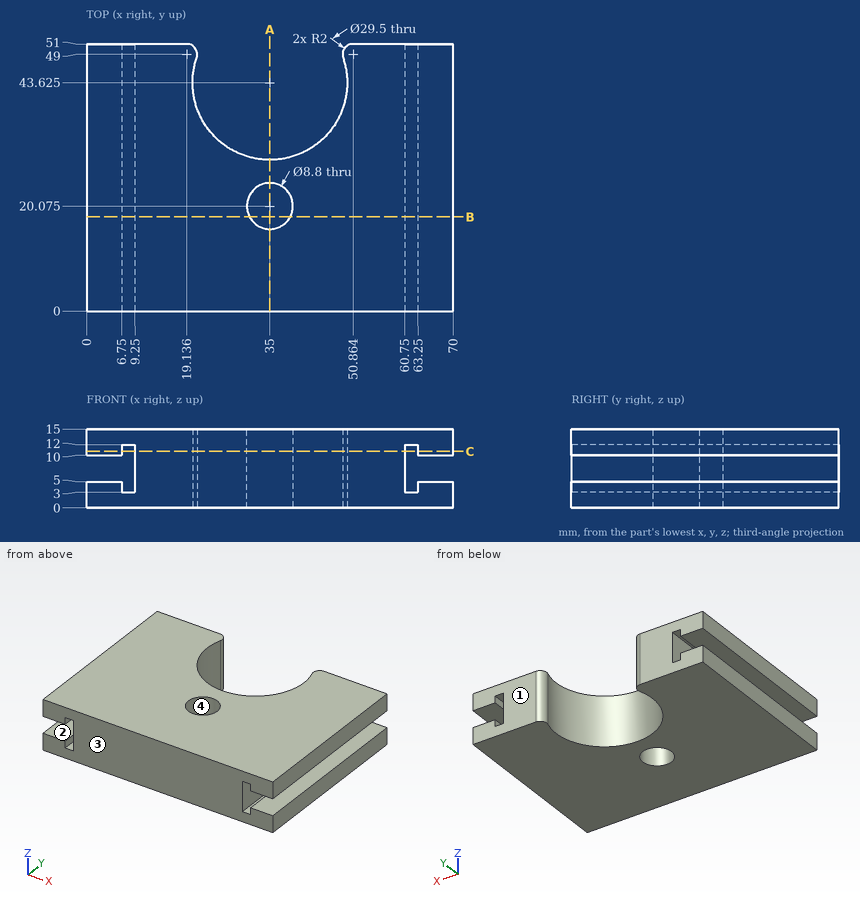
Source: three-view drawing plus pictorial views. Frame: mm from the lowest corner of the part. A direction names the side the tool comes from. Round coordinates to 2 decimals unless told otherwise and drop trailing zeros. Loops run counter-clockwise (first coordinate to the right, second up) from the corner with the lowest first, then second, coordinate; pieces in that order, holes last. Notation, with made-up numbers: M 20.5,-10.5 L 45.5,-10.5 A20 cw 45.5,11.5 Z; hole C 64,-27 d10. An arc over 180 degrees is marked long. Put each result on its own line as item: value.
(1) Ray query, line 1 (Y direction, x = 35, z = 4.5) (3 decimals); line 2 (Z direction, x = 63, y = 39); line 3 (X direction, y = 34.5, z = 3.25). Return the intervals inside material, ascending. Write a range as [from, to].
Solutions:
line 1: [0, 15.675], [24.475, 28.875]
line 2: [0, 3], [12, 15]
line 3: [0, 6.75], [9.25, 23.41], [46.59, 60.75], [63.25, 70]
(2) First-contact query: pin 1 (5 mm diameter, centred on y = 27.5, z = 3.5, fed in from -X). Flat tip, straight axial feed; report the tip coordinate or a pass-through.
Solutions:
pin 1: x = 0
(3) Pull-direction query (X, two-part tool) for the marked faces 3 and 4; classes: released by +X, released by -X, zero draft, split by the parting line, or undercut.
Solutions:
face 3: zero draft
face 4: undercut
(4) Section C-C, the plane z = 10.75. State how many separate pieces and enclosed holes the cut face has, and give its area (3 significant figures).
Solutions:
separate pieces: 3
enclosed holes: 1
area: 2,700 mm²
(5) Section A-A, the plane x = 35. Return loops of the section in (y, z) (3 decimals).
Solutions:
outline: M 0,0 L 15.675,0 L 15.675,15 L 0,15 Z; M 24.475,0 L 28.875,0 L 28.875,15 L 24.475,15 Z
(6) Section B-B, the plane y = 18. Return loops of the section in (x, z), and give its area (3 significant figures).
Solutions:
outline: M 0,0 L 31.12,0 L 31.12,15 L 0,15 L 0,10 L 6.75,10 L 6.75,12 L 9.25,12 L 9.25,3 L 6.75,3 L 6.75,5 L 0,5 Z; M 38.88,0 L 70,0 L 70,5 L 63.25,5 L 63.25,3 L 60.75,3 L 60.75,12 L 63.25,12 L 63.25,10 L 70,10 L 70,15 L 38.88,15 Z
area: 821 mm²
(7) Access query for the marked faces 1 and 2. Directions: +Z, -Z, +X, -X, +Y, -Y. A direction counts if a zero-diameter tool reaches every point of the face in a straight line with its end or side. Return the directions, or none.
Solutions:
face 1: +Z, -Z, +X, -X, +Y
face 2: -X, +Y, -Y
